Geometry: final body of the model. Coordinates: model frame, mm. A direction names the side the tool comes from. Give positions to 0.01 mm unless a question says otherwise; leave off trailing zeros. Write each loop counter-clockwise with the first axis right and the second up, starting at its lowest first coordinate (ties: lowest second). Pieces come first, ordered by that corner, then holes. Notation, with made-up numbers: M -38.5,-37 L -2.5,-37 A12 ccw -2.5,-31 Z; hole C 39,80.25 d2. An arc over 180 degrees is marked long. Answer as a JSON object with one key per item and string values.
from build123d import *

# Parameters (mm, degrees)
SKETCH_1_W          = 60
SKETCH_1_H          = 40
EXTRUDE_1_DEPTH     = 20
SKETCH_2_R          = 10
EXTRUDE_2_DEPTH     = 15
SKETCH_3_W          = 15
SKETCH_3_H          = 5
CUT_EXTRUDE_1_DEPTH = 42.231056256
SKETCH_4_W          = 10
SKETCH_4_H          = 15
CUT_EXTRUDE_2_DEPTH = 73.284161474


with BuildPart() as part:
    # Эскиз1 → Бобышка-Вытянуть1 (new body)
    with BuildSketch(Plane.XY):
        Rectangle(SKETCH_1_W, SKETCH_1_H)
    extrude(amount=EXTRUDE_1_DEPTH)

    # Эскиз2 → Бобышка-Вытянуть2 (add)
    with BuildSketch(Plane.XY.offset(20)):
        with Locations(Location((0, 0, 0), (0, 0, 180))):
            Circle(SKETCH_2_R)
    extrude(amount=EXTRUDE_2_DEPTH)

    # Эскиз3 → Вырез-Вытянуть1 (cut, through all)
    with BuildSketch(Plane.XY.offset(20)):
        with Locations((0, -17.5)):
            Rectangle(SKETCH_3_W, SKETCH_3_H)
    cut_extrude_1 = extrude(amount=-CUT_EXTRUDE_1_DEPTH, mode=Mode.SUBTRACT)

    # Зеркальное отражение1: Вырез-Вытянуть1 across plane
    add(cut_extrude_1.mirror(Plane.ZX), mode=Mode.SUBTRACT)

    # Эскиз4 → Вырез-Вытянуть2 (cut, through all)
    with BuildSketch(Plane.ZY.offset(30)):
        with Locations((5, 0)):
            Rectangle(SKETCH_4_W, SKETCH_4_H)
    extrude(amount=-CUT_EXTRUDE_2_DEPTH, mode=Mode.SUBTRACT)


solid = part.part
1) Cut plane A-A on z = 4. Return loops of the section in (x, y).
Geometry check:
{"outline": "M -30,-20 L -7.5,-20 L -7.5,-15 L 7.5,-15 L 7.5,-20 L 30,-20 L 30,-7.5 L -30,-7.5 Z; M -30,7.5 L 30,7.5 L 30,20 L 7.5,20 L 7.5,15 L -7.5,15 L -7.5,20 L -30,20 Z"}
2) Pull-direction query (Y, two-part tool) for faces 1 (the flat face through (0, -15, 10)), 2 (the flat face through (0, 15, 10)), 3 (the flat face through (0, -7.5, 5)), 4 (the flat face through (-7.5, 18, 10)); classes: pulls with the +Y half, pulls with the -Y half, needs draft (parallel to the pull), parting line crosses it, or undercut.
Geometry check:
{"face 1": "pulls with the -Y half", "face 2": "pulls with the +Y half", "face 3": "undercut", "face 4": "needs draft"}
3) Cut plane C-C on y = 0. Return loops of the section in (x, z), and give its area (3 significant figures).
Geometry check:
{"outline": "M -30,10 L 30,10 L 30,20 L 10,20 L 10,35 L -10,35 L -10,20 L -30,20 Z", "area": "900 mm2"}
4) Cut plane D-D on z = 17. Return loops of the section in (x, y).
Geometry check:
{"outline": "M -30,-20 L -7.5,-20 L -7.5,-15 L 7.5,-15 L 7.5,-20 L 30,-20 L 30,20 L 7.5,20 L 7.5,15 L -7.5,15 L -7.5,20 L -30,20 Z"}
5) Line query: line 1 (Y direction, x = 20.5, z = 4.5); line 2 (X direction, y = 18, z = 15); line 3 (Y direction, x = 3, z = 4.5). Output: solid intervals per line, ascending. Write a range as from..to.
Geometry check:
{"line 1": "y = -20..-7.5, 7.5..20", "line 2": "x = -30..-7.5, 7.5..30", "line 3": "y = -15..-7.5, 7.5..15"}
6) Cut plane B-B on x = -14. Return loops of the section in (y, z), and give its area (3 significant figures).
Geometry check:
{"outline": "M -20,0 L -7.5,0 L -7.5,10 L 7.5,10 L 7.5,0 L 20,0 L 20,20 L -20,20 Z", "area": "650 mm2"}
7) Set-up query: faces 5 (the flat face through (0, 0, 10)), 6 (the flat face through (7.5, -18, 10)), 7 (the cylindrical face through (10, 0, 27)), 8 (the flat face through (0, 14, 0)). Return all of +Z, -Z, +X, -X, +Y, -Y with unobstructed straight access to the full face (end or side cutting, diameter ignored); none if empty.
Geometry check:
{"face 5": "-Z, +X, -X", "face 6": "+Z, -Z, -Y", "face 7": "+Z", "face 8": "-Z, +X, -X, +Y, -Y"}
8) Contact query for flat-ended pins moving along their axis: P1, Ø10, axis at x = 22, y = -12.5, coming from the +Z side; P2, Ø3, axis at x = 5.5, z = 6, coming from the -Y side; P3, Ø4, axis at x = 18, y = 6.5, coming from the -Z side; P4, Ø5, axis at x = -1.5, z = 12, coming from the +Y side. Output: stop coordinate, or through.
Geometry check:
{"P1": "stops at z = 20", "P2": "stops at y = -15", "P3": "stops at z = 0", "P4": "stops at y = 15"}
